Build history of the part. All positions in model axes, mm. Face numbers are marked on the shaded views. A direction names the side the tool comes from. Give positions to 0.01 mm unless a question says otherwise; leave off trailing zeros. Loops run counter-clockwise (first coordinate to the right, second up) from the corner with the lowest first, then second, coordinate; pieces in that order, holes last. Notation, with made-up numbers: M 13.5,84 L 25.5,84 A8 ccw 25.5,99 Z; hole C 46.25,34 d9. An arc over 180 degrees is marked long. Answer in a Markdown table with one row per item. Add a question column.
```python
from build123d import *

# Parameters (mm, degrees)
SKETCH_1_R          = 1.25
SKETCH_1_R_2        = 13.5
EXTRUDE_1_DEPTH     = 5
SKETCH_2_R          = 2.75
CUT_EXTRUDE_1_DEPTH = 1
SKETCH_4_W          = 34
SKETCH_4_H          = 59
CUT_EXTRUDE_3_DEPTH = 2
EXTRUDE_2_DEPTH     = 3
CHAMFER_1_SIZE      = 2
CUT_EXTRUDE_4_DEPTH = 1.5
FILLET_3_R          = 1


with BuildPart() as part:
    # 草图1 → 凸台-拉伸1 (new body)
    with BuildSketch(Plane.XY):
        with BuildLine():
            Line((-16.75, -16.75), (-16.75, -44.75))
            Line((-16.75, -44.75), (16.75, -44.75))
            Line((16.75, -44.75), (16.75, -19.75))
            Line((16.75, -19.75), (19.75, -17.232701106))
            Line((19.75, -17.232701106), (19.75, 0))
            ThreePointArc((19.75, 0), (0, 19.75), (-19.75, 0))
            Line((-19.75, 0), (-19.75, -13.75))
            Line((-19.75, -13.75), (-16.75, -16.75))
        make_face()
        with Locations((-13.5, -41.5)):
            Circle(SKETCH_1_R, mode=Mode.SUBTRACT)
        with Locations((13.5, -41.5)):
            Circle(SKETCH_1_R, mode=Mode.SUBTRACT)
        Circle(SKETCH_1_R_2, mode=Mode.SUBTRACT)
        with Locations((-13.5, 10.5)):
            Circle(SKETCH_1_R, mode=Mode.SUBTRACT)
        with Locations((13.5, 10.5)):
            Circle(SKETCH_1_R, mode=Mode.SUBTRACT)
    extrude(amount=EXTRUDE_1_DEPTH)

    # 草图2 → 切除-拉伸1 (cut)
    with BuildSketch(Plane(origin=(0, 0, 0), x_dir=(-1, 0, 0), z_dir=(0, 0, -1))):
        with Locations((-13.5, -41.5)):
            Circle(SKETCH_2_R)
        with Locations((13.5, -41.5)):
            Circle(SKETCH_2_R)
    extrude(amount=-CUT_EXTRUDE_1_DEPTH, mode=Mode.SUBTRACT)

    # 草图4 → 切除-拉伸3 (cut)
    with BuildSketch(Plane.XY.offset(5)):
        with Locations((0, -15.25)):
            Rectangle(SKETCH_4_W, SKETCH_4_H)
    extrude(amount=-CUT_EXTRUDE_3_DEPTH, mode=Mode.SUBTRACT)

    # 草图5 → 凸台-拉伸2 (add)
    with BuildSketch(Plane(origin=(0, 0, 0), x_dir=(-1, 0, 0), z_dir=(0, 0, -1))):
        with BuildLine():
            Line((-16.75, -22), (13.75, -22))
            Line((13.75, -22), (16.75, -19))
            Line((16.75, -19), (16.75, -16.75))
            Line((16.75, -16.75), (19.75, -13.75))
            Line((19.75, -13.75), (19.75, -7.341092536))
            Line((19.75, -7.341092536), (11.300756088, -11.281039678))
            Line((11.300756088, -11.281039678), (7.165897883, -15.415897883))
            ThreePointArc((7.165897883, -15.415897883), (-0.466019686, -16.993611319), (-8, -15))
            Line((-8, -15), (-19.75, -15))
            Line((-19.75, -15), (-19.75, -17.232701106))
            Line((-19.75, -17.232701106), (-16.75, -19.75))
            Line((-16.75, -19.75), (-16.75, -22))
        make_face()
    extrude(amount=EXTRUDE_2_DEPTH)

    # 倒角1
    chamfer_1_edges = [part.edges().sort_by_distance(p)[0] for p in [
        (1.5, -22, -3),
        (-15.25, -20.5, -3),
    ]]
    chamfer(chamfer_1_edges, length=CHAMFER_1_SIZE)

    # 草图8 → 切除-拉伸4 (cut)
    with BuildSketch(Plane(origin=(0, 0, 0), x_dir=(-1, 0, 0), z_dir=(0, 0, -1))):
        with BuildLine():
            Line((-19.75, -15), (-8, -15))
            ThreePointArc((-8, -15), (-0.466019686, -16.993611319), (7.165897883, -15.415897883))
            Line((7.165897883, -15.415897883), (11.300756088, -11.281039678))
            Line((11.300756088, -11.281039678), (19.75, -7.341092536))
            Line((19.75, -7.341092536), (19.75, 0))
            ThreePointArc((19.75, 0), (0, 19.75), (-19.75, 0))
            Line((-19.75, 0), (-19.75, -15))
        make_face()
    extrude(amount=-CUT_EXTRUDE_4_DEPTH, mode=Mode.SUBTRACT)

    # 圆角3
    fillet_3_edges = [part.edges().sort_by_distance(p)[0] for p in [
        (16.75, -44.75, 1.5),
        (-16.75, -44.75, 1.5),
    ]]
    fillet(fillet_3_edges, radius=FILLET_3_R)


solid = part.part
```
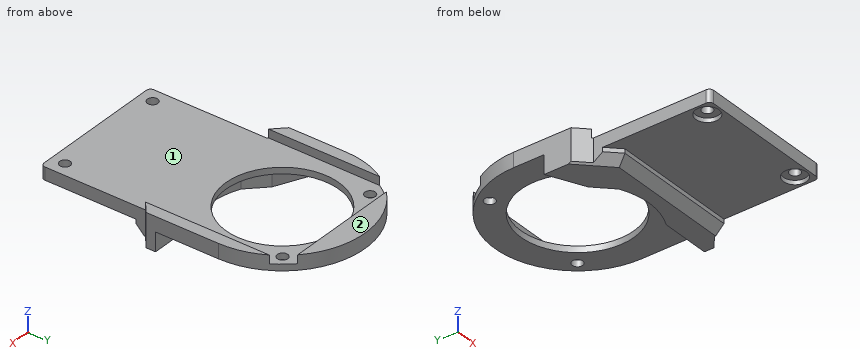
(1) Slice it at D-D, the plane y = -31. Give the cut face in (x, z).
(2) Pin check, flat tips, straight feed: pin 1 (1.3 mm diameter, centred on x = 15, z = -1.5, fed in from +Y); pin 2 (1.6 mm diameter, centred on x = -13.5, y = -41, fed in from -Z); pin 3 (6 mm diameter, centred on x = -13, y = -1, fed in from -Z). Stop position of each tip, or through.
(3) Slice it at C-C, the plane x = 6. Give the cut face in (y, z), then the cut area to 3 significant figures.
(4) Wall check: line 1 (X direction, y = -41.5, z = 1.95); line 2 (Y direction, x = 13.5, z = 0.25); line 3 (X direction, y = 10.5, z = 2.6). Give the ranges that are in metal, low to high.
(5) Slice it at B-B, the plane z = 4. Give the cut face in (x, y), then the cut area to 3 significant figures.
(6) Tool access for the marked faces 1 and 2: list every direction of +Z, -Z, +X, -X, +Y, -Y with a clear straight run to the whole face (end or side of a thin tool).
(7) Slice it at A-A, the plane x = 0. Give the cut face in (y, z).
Solution:
| question | item | result |
|---|---|---|
| 1 | outline | M -16.75,0 L 16.75,0 L 16.75,3 L -16.75,3 Z |
| 2 | pin 1 | y = -15 |
| 2 | pin 2 | z = 1 |
| 2 | pin 3 | z = 1.5 |
| 3 | outline | M -44.75,0 L -22,0 L -22,-1 L -20,-3 L -15.91,-3 L -15.91,1.5 L -12.09,1.5 L -12.09,3 L -44.75,3 Z; M 12.09,1.5 L 18.82,1.5 L 18.82,5 L 14.25,5 L 14.25,3 L 12.09,3 Z |
| 3 | area | 128 mm^2 |
| 4 | line 1 | -16.75 to -14.75, -12.25 to 12.25, 14.75 to 16.75 |
| 4 | line 2 | -44.75 to -44.25, -38.75 to -15 |
| 4 | line 3 | -16.73 to -14.75, -12.25 to -8.49, 8.49 to 12.25, 14.75 to 16.73 |
| 5 | outline | M -19.75,-13.75 L -17,-16.5 L -17,10.05 A19.75 ccw -19.75,0 Z; M -13.67,14.25 L 13.67,14.25 A19.75 ccw Z; M 17,-19.54 L 19.75,-17.23 L 19.75,0 A19.75 ccw 17,10.05 Z |
| 5 | area | 233 mm^2 |
| 6 | face 1 | +Z, -Y |
| 6 | face 2 | +Z, +X, -X, +Y, -Y |
| 7 | outline | M -44.75,0 L -22,0 L -22,-1 L -20,-3 L -17,-3 L -17,1.5 L -13.5,1.5 L -13.5,3 L -44.75,3 Z; M 13.5,1.5 L 19.75,1.5 L 19.75,5 L 14.25,5 L 14.25,3 L 13.5,3 Z |
